Geometry: final body of the model. Coordinates: model frame, mm. Coordinates: 2 decimals unless noted, no trailing zeros. Order: outer loops, then holes, each group sorted by start corner. A loop starts at its lowest first (then second) coordinate and runs counter-clockwise, first axis right, second up. Notation, with made-up numbers: M -15.5,-9.5 L 20.5,-9.5 A28 ccw 20.5,15.5 Z; hole C 19.25,8.5 d1. An arc over 180 degrees is marked long. Use CSV: the item, a comma, the result in double quotes. Start each with the question number.
Q1. Section query A-A, the plane x = -34. Output: boundary loops of the cut face in (y, z) (3 decimals), and give its area (3 significant figures).
Q2. Ray query, probe 1 along X at (y, z) = (0.8, 51.75); probe 2 along X at (y, z) = (3.15, 51); probe 3 along X at (y, z) = (4, 51.75). Return the intervals inside material, ascending.
Q3. Section query B-B, the plane y = 0.75. Output: boundary loops of the cut face in (x, z), and give its area (3 significant figures).
Q4. Section query C-C, the plane x = 20.5. Output: boundary loops of the cut face in (y, z), and give its area (3 significant figures).
Q5. First-contact query: P1, Ø1, axis at x = 22.5, y = 3.5, coming from the -Z side; P2, Ø2, axis at x = 49, z = 57.5, coming from the +Y side; P3, Ø2, axis at y = 4, z = 56, coming from the -X side; P4, Ø1.4, axis at y = 4.5, z = 46.5, coming from the -X side. Flat tips, straight axial feed; report the tip coordinate or a pass-through.
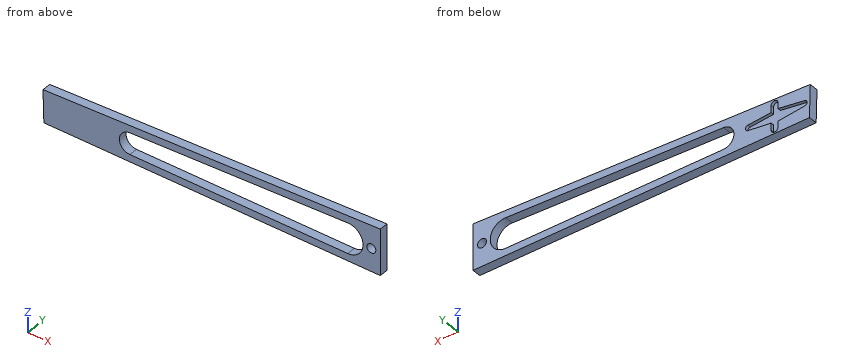
from build123d import *

# Parameters (mm, degrees)
SKETCH1_R           = 2.5
BOSS_EXTRUDE1_DEPTH = 5
BOSS_EXTRUDE2_DEPTH = 3.2


with BuildPart() as part:
    # Sketch1 → Boss-Extrude1 (new body)
    with BuildSketch(Plane(origin=(0, 0, 0), x_dir=(1, 0, 0), z_dir=(0, 1, 0))):
        Polygon((-90.005103209, -41.999399148), (-90.480022259, -59.993132832), (97.6446575, -63.815482804), (97.6446575, -38.32994317), align=None)
        with Locations((92.6446575, -51.070678602)):
            Circle(SKETCH1_R, mode=Mode.SUBTRACT)
        with BuildLine():
            Line((79.480798132, -42.685898751), (-42.056384532, -45.062535629))
            ThreePointArc((-42.056384532, -45.062535629), (-47.894488465, -51.013496449), (-42.061229083, -56.969206079))
            Line((-42.061229083, -56.969206079), (79.473979342, -59.444743533))
            ThreePointArc((79.473979342, -59.444743533), (88.025749222, -51.068799274), (79.480798132, -42.685898751))
        make_face(mode=Mode.SUBTRACT)
        with BuildLine():
            Line((-72.450254412, -44.247483492), (-72.450254412, -47.547483492))
            Line((-72.450254412, -47.547483492), (-87.444932153, -49.510170284))
            ThreePointArc((-87.444932153, -49.510170284), (-88.750254412, -50.997483492), (-87.444932153, -52.484796699))
            Line((-87.444932153, -52.484796699), (-72.450254412, -54.447483492))
            Line((-72.450254412, -54.447483492), (-72.450254412, -57.747483492))
            ThreePointArc((-72.450254412, -57.747483492), (-70.550254412, -59.647483492), (-68.650254412, -57.747483492))
            Line((-68.650254412, -57.747483492), (-68.650254412, -53.897483492))
            Line((-68.650254412, -53.897483492), (-55.640888759, -52.509143053))
            ThreePointArc((-55.640888759, -52.509143053), (-54.299665811, -51.008287292), (-55.644843725, -49.510975235))
            Line((-55.644843725, -49.510975235), (-68.650254412, -48.097483492))
            Line((-68.650254412, -48.097483492), (-68.650254412, -44.247483492))
            ThreePointArc((-68.650254412, -44.247483492), (-70.550254412, -42.347483492), (-72.450254412, -44.247483492))
        make_face(mode=Mode.SUBTRACT)
    extrude(amount=BOSS_EXTRUDE1_DEPTH)

    # Sketch1_16 → Boss-Extrude2 (add)
    with BuildSketch(Plane(origin=(0, 0, 0), x_dir=(1, 0, 0), z_dir=(0, 1, 0))):
        with BuildLine():
            Line((-72.450254412, -44.247483492), (-72.450254412, -47.547483492))
            Line((-72.450254412, -47.547483492), (-87.444932153, -49.510170284))
            ThreePointArc((-87.444932153, -49.510170284), (-88.750254412, -50.997483492), (-87.444932153, -52.484796699))
            Line((-87.444932153, -52.484796699), (-72.450254412, -54.447483492))
            Line((-72.450254412, -54.447483492), (-72.450254412, -57.747483492))
            ThreePointArc((-72.450254412, -57.747483492), (-70.550254412, -59.647483492), (-68.650254412, -57.747483492))
            Line((-68.650254412, -57.747483492), (-68.650254412, -53.897483492))
            Line((-68.650254412, -53.897483492), (-55.640888759, -52.509143053))
            ThreePointArc((-55.640888759, -52.509143053), (-54.299665811, -51.008287292), (-55.644843725, -49.510975235))
            Line((-55.644843725, -49.510975235), (-68.650254412, -48.097483492))
            Line((-68.650254412, -48.097483492), (-68.650254412, -44.247483492))
            ThreePointArc((-68.650254412, -44.247483492), (-70.550254412, -42.347483492), (-72.450254412, -44.247483492))
        make_face()
    extrude(amount=BOSS_EXTRUDE2_DEPTH)


solid = part.part
Responses:
1,outline,"M 0,40.904 L 5,40.904 L 5,44.905 L 0,44.905 Z; M 0,57.133 L 5,57.133 L 5,61.141 L 0,61.141 Z"
1,area,"40.0 mm²"
2,probe 1,"x = -90.26 to -47.85, 88 to 90.24, 95.05 to 97.64"
2,probe 2,"x = -90.24 to -47.89, 88.03 to 90.15, 95.14 to 97.64"
2,probe 3,"x = -90.26 to -88.55, -54.49 to -47.85, 88 to 90.24, 95.05 to 97.64"
3,outline,"M -90.48,59.99 L -90.01,42 L 97.64,38.33 L 97.64,63.82 Z; hole M -42.06,45.06 L 79.48,42.69 A8.38 ccw long 79.47,59.44 L -42.06,56.97 A5.95 ccw Z; hole C 92.64,51.07 d5"
3,area,"2,160 mm²"
4,outline,"M 0,39.84 L 5,39.84 L 5,43.84 L 0,43.84 Z; M 0,58.24 L 5,58.24 L 5,62.25 L 0,62.25 Z"
4,area,"40.0 mm²"
5,P1,"stops at z = 39.79"
5,P2,"passes through"
5,P3,"stops at x = -90.4"
5,P4,"stops at x = -90.14"
